Answer from the drawing. Dimensions are ordinates in mm from the lowest x, y and z of the part. Round coordinates to 2 decimals unless told otherwise and drop trailing zeros. Write each loop counter-clockwise with the first axis right and the second up, starting at its lowest first coordinate (ties: lowest second). Pieces come first, ordered by that corner, then holes. Notation, with made-up numbers: (5.5, 53) -> (45.5, 53) arc R23 cw to (45.5, 70) -> close; hole circle Ø3 at (14.25, 7). An arc over 180 degrees is marked (long way). Return JSON: item names as keys, results as strings. Group by question number.
(1) Straight lines are drawn through the part: line 1 (Y direction, x = 31.5, z = 0.95); line 2 (Y direction, x = 38, z = 3.3); line 3 (X direction, y = 33.5, z = 2.75). For each, find the intervals that lie inside material, in ascending order.
(2) A cutting plane is placed at B-B on z = 2.95. Give the vertices of the cut face in (x, y), then the cut area to 3 significant figures.
(3) Given pin 1 (8 mm diameter, centred on x = 72, y = 16, fed in from -Z); pin 2 (2.5 mm diameter, centred on x = 41.5, z = 2, fed in from +Y); pin 3 (1.5 mm diameter, centred on x = 55.5, z = 2.5, fed in from -Y); pin 4 (2 mm diameter, centred on x = 81, z = 3.5, fed in from -Y), each flat-ended and moving along its own axis, determine where each tip first touches the part or whether it passes through.
(4) A cutting plane is placed at D-D on y = 104. Give the vertices of the cut face in (x, z).
(5) A cutting plane is placed at A-A on x = 60. Give the vertices of the cut face in (y, z), then the cut area to 3 significant figures.
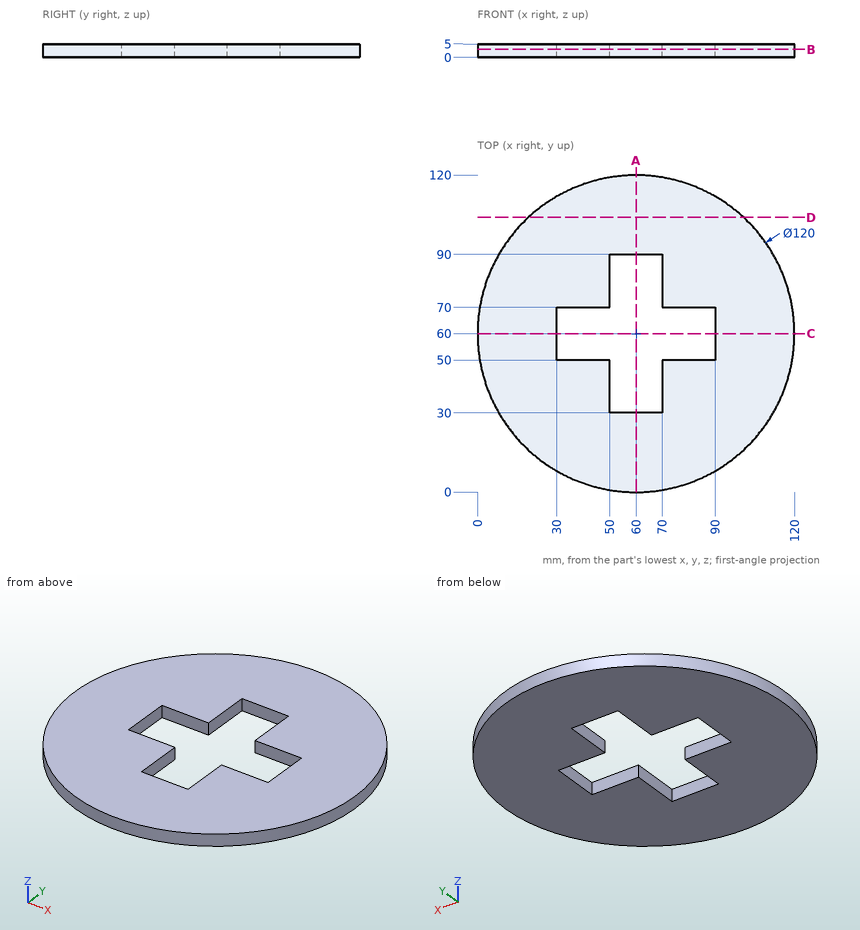
Checks:
{
 "1": {"line 1": "y = 7.2 to 50, 70 to 112.8", "line 2": "y = 4.18 to 50, 70 to 115.82", "line 3": "x = 6.17 to 50, 70 to 113.83"},
 "2": {"outline": "circle Ø120 at (60, 60); hole (30, 50) -> (50, 50) -> (50, 30) -> (70, 30) -> (70, 50) -> (90, 50) -> (90, 70) -> (70, 70) -> (70, 90) -> (50, 90) -> (50, 70) -> (30, 70) -> close", "area": "9,310 mm^2"},
 "3": {"pin 1": "stops at z = 0", "pin 2": "stops at y = 117.47", "pin 3": "stops at y = 0.12", "pin 4": "stops at y = 3.43"},
 "4": {"outline": "(19.21, 0) -> (100.79, 0) -> (100.79, 5) -> (19.21, 5) -> close"},
 "5": {"outline": "(0, 0) -> (30, 0) -> (30, 5) -> (0, 5) -> close; (90, 0) -> (120, 0) -> (120, 5) -> (90, 5) -> close", "area": "300 mm^2"}
}
